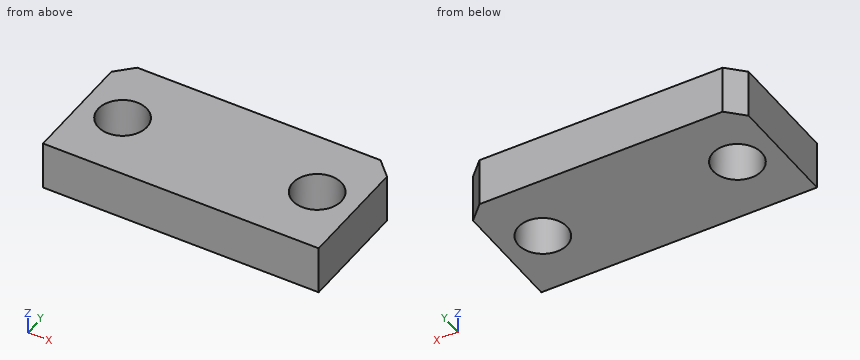
```python
from build123d import *

# Parameters (mm, degrees)
ESQUISSE1_W        = 17
ESQUISSE1_H        = 8
ESQUISSE1_R        = 1.5
BOSS_EXTRU_1_DEPTH = 3
CHANFREIN1_SIZE    = 1


with BuildPart() as part:
    # Esquisse1 → Boss.-Extru.1 (new body)
    with BuildSketch(Plane.XY):
        Rectangle(ESQUISSE1_W, ESQUISSE1_H)
        with Locations((-6, 0)):
            Circle(ESQUISSE1_R, mode=Mode.SUBTRACT)
        with Locations((6, 0)):
            Circle(ESQUISSE1_R, mode=Mode.SUBTRACT)
    extrude(amount=BOSS_EXTRU_1_DEPTH)

    # Chanfrein1
    chanfrein1_edges = [part.edges().sort_by_distance(p)[0] for p in [
        (-8.5, 4, 1.5),
        (8.5, 4, 1.5),
    ]]
    chamfer(chanfrein1_edges, length=CHANFREIN1_SIZE)


solid = part.part
```
Input: part model. Units: mm. Frame: model coordinates. Give positions to 0.01 mm unless a question says otherwise; leave off trailing zeros. Order: outer loops, then holes, each group sorted by start corner. A loop starts at its lowest first (then second) coordinate and runs counter-clockwise, first axis right, second up. Notation, with made-up numbers: (1.5, -6.5) - (35.5, -6.5) arc R22 ccw to (35.5, 1.5) - close; hole circle Ø8 at (-20, -28.75). An arc over 180 degrees is marked (long way). Use a Markdown table: item, result.
(1) Pin query (flat end, axial travel): pin 1 (1 mm diameter, centred on x = 6.5, y = -3, fed in from -Z). Return the tip coordinate at first contact, or that it passes through.
Computed values:
| item | result |
|---|---|
| pin 1 | stops at z = 0 |
(2) Section query B-B (y = 0). Output: boundary loops of the cut face in (x, z).
Computed values:
| item | result |
|---|---|
| outline | (-8.5, 0) - (-7.5, 0) - (-7.5, 3) - (-8.5, 3) - close; (-4.5, 0) - (4.5, 0) - (4.5, 3) - (-4.5, 3) - close; (7.5, 0) - (8.5, 0) - (8.5, 3) - (7.5, 3) - close |
(3) Line query: line 1 (Y direction, x = 6, z = 1.75); line 2 (X direction, y = -1.25, z = 0.5); line 3 (X direction, y = 0.5, z = 2.55). Output: solid intervals per line, ascending. Write a range as from..to.
Computed values:
| item | result |
|---|---|
| line 1 | y = -4..-1.5, 1.5..4 |
| line 2 | x = -8.5..-6.83, -5.17..5.17, 6.83..8.5 |
| line 3 | x = -8.5..-7.41, -4.59..4.59, 7.41..8.5 |
(4) Section query A-A (z = 0.25). Output: boundary loops of the cut face in (x, y).
Computed values:
| item | result |
|---|---|
| outline | (-8.5, -4) - (8.5, -4) - (8.5, 3) - (7.5, 4) - (-7.5, 4) - (-8.5, 3) - close; hole circle Ø3 at (-6, 0); hole circle Ø3 at (6, 0) |
(5) Section query D-D (y = -1). Output: boundary loops of the cut face in (x, z).
Computed values:
| item | result |
|---|---|
| outline | (-8.5, 0) - (-7.12, 0) - (-7.12, 3) - (-8.5, 3) - close; (-4.88, 0) - (4.88, 0) - (4.88, 3) - (-4.88, 3) - close; (7.12, 0) - (8.5, 0) - (8.5, 3) - (7.12, 3) - close |
(6) Section query C-C (x = -6). Output: boundary loops of the cut face in (y, z).
Computed values:
| item | result |
|---|---|
| outline | (-4, 0) - (-1.5, 0) - (-1.5, 3) - (-4, 3) - close; (1.5, 0) - (4, 0) - (4, 3) - (1.5, 3) - close |
